Check sheet for the modelled part. Datum: model origin and axes. Units: mm. A direction names the side the tool comes from. Round coordinates to 2 decimals unless told otherwise and drop trailing zeros. Loops run counter-clockwise (first coordinate to the right, second up) from the corner with the lowest first, then second, coordinate; pieces in that order, holes last. Notation, with made-up numbers: (32.25, 9.5) -> (48.25, 9.5) arc R14 ccw to (48.25, 14.5) -> close; hole circle Ø1 at (-2.5, 88.5). An arc over 180 degrees is marked (long way). Use one line per item in the form item = value. Start each with the question number.
(1) Set-up check for faces 4 (the cylindrical face through (271.16, 355.45, 83.59)), 5 (the cylindrical face through (343.34, 301.52, 5.07)): record each of +Z, -Z, +X, -X, +Y, -Y from which the full face is reachable in a straight line by a thin tool's end or side.
(2) Sectioned sample at D-D (x = 239.5). Record the cut outline in (y, z).
(3) Sectioned sample at C-C (z = 97). Record the cut outline in (x, y).
(4) Material ranges on probe 1 along X at (y, z) = (300, 68.5); probe 2 along Z at (x, y) = (253.5, 262.5), recorded low to high. Write a range as [from, to].
(5) Draft check along X on faces 1 (the flat face through (299, 284, 10)), 2 (the cylindrical face through (343.34, 301.52, 84.41)), 3 (the cylindrical face through (305.723, 301.802, 32.185)). Enter one of: released by +X, released by -X, zero draft, split by the parting line, or undercut.
(6) Sectioned sample at B-B (y = 255). Record the cut outline in (x, z), and give its area (3 significant figures).
(7) Go/stop test with flat-tipped pins: pin 1 (5 mm diameter, centred on x = 255.5, z = 58, fed in from -Y); pin 2 (3 mm diameter, centred on x = 326.5, z = 62.5, fed in from -Y); pin 3 (1.5 mm diameter, centred on x = 247, y = 337, fed in from +Z). Record where each tip stops, or that it passes through.
(8) Sectioned sample at A-A (x = 300). Record the cut outline in (y, z).
from build123d import *

# Parameters (mm, degrees)
SKETCH1_R           = 62.5
BOSS_EXTRUDE1_DEPTH = 58
SKETCH2_R           = 6
BOSS_EXTRUDE2_DEPTH = 113
SKETCH3_R           = 75
BOSS_EXTRUDE3_DEPTH = 10
SKETCH4_R           = 2.25
CUT_EXTRUDE1_DEPTH  = 133
SKETCH5_R           = 2.25
CUT_EXTRUDE2_DEPTH  = 133
SKETCH6_R           = 2.25
CUT_EXTRUDE3_DEPTH  = 133
SKETCH7_R           = 2.25
CUT_EXTRUDE4_DEPTH  = 133


with BuildPart() as part:
    # Sketch1 → Boss-Extrude1 (new body)
    with BuildSketch(Plane.XY.offset(55)):
        with Locations(Location((300, 300, 0), (0, 0, 180))):
            Circle(SKETCH1_R)
    extrude(amount=BOSS_EXTRUDE1_DEPTH)

    # Sketch2 → Boss-Extrude2 (add)
    with BuildSketch(Plane.XY):
        with Locations((300, 300)):
            Circle(SKETCH2_R)
    extrude(amount=BOSS_EXTRUDE2_DEPTH)

    # Sketch3 → Boss-Extrude3 (add)
    with BuildSketch(Plane.XY):
        with Locations((300, 300)):
            Circle(SKETCH3_R)
    extrude(amount=BOSS_EXTRUDE3_DEPTH)

    # Sketch4 → Cut-Extrude1 (cut)
    with BuildSketch(Plane.XY.offset(113)):
        with Locations((345, 300)):
            Circle(SKETCH4_R)
    extrude(amount=-CUT_EXTRUDE1_DEPTH, mode=Mode.SUBTRACT)

    # Sketch5 → Cut-Extrude2 (cut)
    with BuildSketch(Plane.XY.offset(113)):
        with Locations((255, 300)):
            Circle(SKETCH5_R)
    extrude(amount=-CUT_EXTRUDE2_DEPTH, mode=Mode.SUBTRACT)

    # Sketch6 → Cut-Extrude3 (cut)
    with BuildSketch(Plane.XY.offset(113)):
        with Locations((300, 345)):
            Circle(SKETCH6_R)
    extrude(amount=-CUT_EXTRUDE3_DEPTH, mode=Mode.SUBTRACT)

    # Sketch7 → Cut-Extrude4 (cut)
    with BuildSketch(Plane.XY.offset(113)):
        with Locations((300, 255)):
            Circle(SKETCH7_R)
    extrude(amount=-CUT_EXTRUDE4_DEPTH, mode=Mode.SUBTRACT)


solid = part.part
Checks:
q1.face_4 = +Z
q1.face_5 = +Z, -Z
q2.outline = (255.67, 0) -> (344.33, 0) -> (344.33, 10) -> (255.67, 10) -> close; (284.32, 55) -> (315.68, 55) -> (315.68, 113) -> (284.32, 113) -> close
q3.outline = circle Ø125 at (300, 300); hole circle Ø4.5 at (255, 300); hole circle Ø4.5 at (300, 255); hole circle Ø4.5 at (300, 345); hole circle Ø4.5 at (345, 300)
q4.probe_1 = [237.5, 252.75], [257.25, 342.75], [347.25, 362.5]
q4.probe_2 = [0, 10], [55, 113]
q5.face_1 = zero draft
q5.face_2 = undercut
q5.face_3 = split by the parting line
q6.outline = (240, 0) -> (297.75, 0) -> (297.75, 10) -> (240, 10) -> close; (256.63, 55) -> (297.75, 55) -> (297.75, 113) -> (256.63, 113) -> close; (302.25, 0) -> (360, 0) -> (360, 10) -> (302.25, 10) -> close; (302.25, 55) -> (343.37, 55) -> (343.37, 113) -> (302.25, 113) -> close
q6.area = 5,930 mm2
q7.pin_1 = 253.72
q7.pin_2 = 242.72
q7.pin_3 = 10
q8.outline = (225, 0) -> (252.75, 0) -> (252.75, 10) -> (225, 10) -> close; (237.5, 55) -> (252.75, 55) -> (252.75, 113) -> (237.5, 113) -> close; (257.25, 0) -> (342.75, 0) -> (342.75, 10) -> (306, 10) -> (306, 55) -> (342.75, 55) -> (342.75, 113) -> (257.25, 113) -> (257.25, 55) -> (294, 55) -> (294, 10) -> (257.25, 10) -> close; (347.25, 0) -> (375, 0) -> (375, 10) -> (347.25, 10) -> close; (347.25, 55) -> (362.5, 55) -> (362.5, 113) -> (347.25, 113) -> close
